Model file for the job. Use its own axes, mm. Face numbers are marked on the shaded views. Give positions to 0.01 mm unless a question says otherwise; leave off trailing zeros. Loops run counter-clockwise (first coordinate to the right, second up) from the corner with the lowest first, then second, coordinate; pieces in that order, holes last. Notation, with made-up numbers: (64.25, -15) - (108.25, -15) arc R14 ccw to (108.25, 7) - close; hole circle Ø9 at (5, -26). An arc over 180 degrees is marked (long way). Answer as CSV lines item,"result". Start each with the question number.
Item 1: Pull direction X, two halves, no side cores. Call the marked faces 1, 2 and 3: pulls with the +X half, pulls with the -X half, needs draft (parallel to the pull), parting line crosses it, or undercut.
Item 2: Saw through at C-C on y = 2. Give the cut face in (x, z).
Item 3: Saw through at B-B on z = -18. Give the cut face in (x, y).
Item 4: Drill centre lines: L1, parallel to X at y = 4.25, z = 0; L2, parallel to Z at x = -12, y = 5.75; L3, parallel to Z at x = -5.5, y = 3. Where is each one in solid material? Low to high. Write a range as from..to.
Item 5: Saw through at D-D on z = 3. Give the cut face in (x, y).
Item 6: Saw through at A-A on x = 11.3. Give the cut face in (y, z).
Item 7: Pin check, flat tips, straight feed: pin 1 (4 mm diameter, centred on y = 5, z = -9, fed in from -X); pin 2 (1.5 mm diameter, centred on x = -5.5, z = 17, fed in from -Y); pin 3 (3 mm diameter, centred on y = 5, z = -9, fed in from -X); pin 4 (4.5 mm diameter, centred on y = 5, z = 9, fed in from -X). Stop position of each tip, or through.
from build123d import *

# Parameters (mm, degrees)
SKETCH_1_W          = 32.7
SKETCH_1_H          = 51
EXTRUDE_1_DEPTH     = 12
SKETCH_2_R          = 2.6
SKETCH_2_R_2        = 1.6
CUT_EXTRUDE_1_DEPTH = 33.581781719
SKETCH_3_W          = 10
SKETCH_3_H          = 2
CUT_EXTRUDE_2_DEPTH = 55.884628996


# Read off the part's stored shape, not the designer's step: 高级异型孔1
with BuildPart() as part:
    # 草图1 → 凸台-拉伸1 (new body)
    with BuildSketch(Plane(origin=(0, 0, 0), x_dir=(1, 0, 0), z_dir=(0, 1, 0))):
        Rectangle(SKETCH_1_W, SKETCH_1_H)
    extrude(amount=EXTRUDE_1_DEPTH)

    # 草图2 → 切除-拉伸1 (cut, through all)
    with BuildSketch(Plane(origin=(0, 12, 0), x_dir=(1, 0, 0), z_dir=(0, 1, 0))):
        with Locations(Location((-11.3, 18, 0), (0, 0, 270))):
            Circle(SKETCH_2_R)
        with Locations(Location((11.3, 18, 0), (0, 0, 90))):
            Circle(SKETCH_2_R)
        with Locations(Location((11.3, -18, 0), (0, 0, 270))):
            Circle(SKETCH_2_R)
        with Locations(Location((-11.3, -18, 0), (0, 0, 90))):
            Circle(SKETCH_2_R)
        with Locations(Location((11.3, 0, 0), (0, 0, 270))):
            Circle(SKETCH_2_R_2)
        with Locations(Location((-11.3, 0, 0), (0, 0, 90))):
            Circle(SKETCH_2_R_2)
    extrude(amount=-CUT_EXTRUDE_1_DEPTH, mode=Mode.SUBTRACT)

    # 草图3 → 切除-拉伸2 (cut, through all)
    with BuildSketch(Plane.XY.offset(25.5)):
        with Locations((0, 11)):
            Rectangle(SKETCH_3_W, SKETCH_3_H)
    extrude(amount=-CUT_EXTRUDE_2_DEPTH, mode=Mode.SUBTRACT)

    # 高级异型孔1 outline → 高级异型孔1 (revolve, cut)
    with BuildSketch(Plane(origin=(0, 5, 9), x_dir=(0, 1, 0), z_dir=(0, 0, -1))):
        Polygon((3.6, -16.35), (3.6, -15.35), (2.3, -15.35), (2.3, -5.35), (0, -3.96802058), (0, -16.35), align=None)
    other_1 = revolve(axis=Axis((0, 5, 9), (1, 0, 0)), mode=Mode.SUBTRACT)

    # Other 1 2 outline → Other 1 2 (revolve, cut)
    with BuildSketch(Plane(origin=(0, 5, -9), x_dir=(0, 1, 0), z_dir=(0, 0, -1))):
        Polygon((0, -16.35), (3.6, -16.35), (3.6, -15.35), (2.3, -15.35), (2.3, -5.35), (0, -3.96802058), align=None)
    other_1_2 = revolve(axis=Axis((0, 5, -9), (1, 0, 0)), mode=Mode.SUBTRACT)

    # 镜向1: 高级异型孔1, Other 1 2 across plane
    add(other_1.mirror(Plane(origin=(0, 0, 0), x_dir=(0, 0, 1), z_dir=(1, 0, 0))), mode=Mode.SUBTRACT)
    add(other_1_2.mirror(Plane(origin=(0, 0, 0), x_dir=(0, 0, 1), z_dir=(1, 0, 0))), mode=Mode.SUBTRACT)


solid = part.part
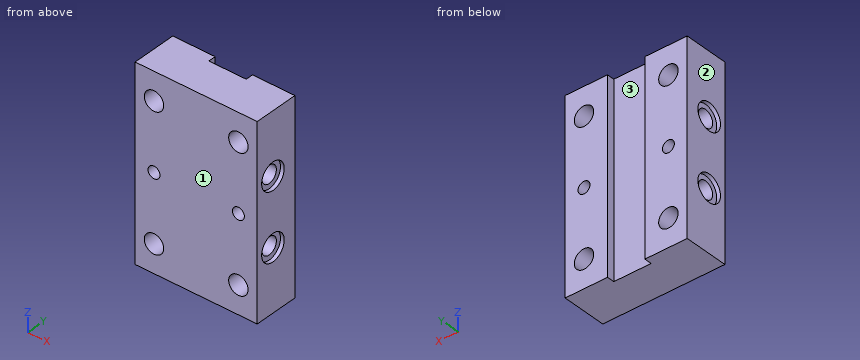
Responses:
1,face 1,"needs draft"
1,face 2,"pulls with the -X half"
1,face 3,"undercut"
2,outline,"(-16.35, -25.5) - (16.35, -25.5) - (16.35, -10.99) - (15.35, -10.99) - (15.35, -7.01) - (16.35, -7.01) - (16.35, 7.01) - (15.35, 7.01) - (15.35, 10.99) - (16.35, 10.99) - (16.35, 25.5) - (-16.35, 25.5) - (-16.35, 10.99) - (-15.35, 10.99) - (-15.35, 7.01) - (-16.35, 7.01) - (-16.35, -7.01) - (-15.35, -7.01) - (-15.35, -10.99) - (-16.35, -10.99) - close; hole circle Ø5.2 at (-11.3, -18); hole circle Ø5.2 at (-11.3, 18); hole circle Ø3.2 at (-11.3, 0); hole circle Ø5.2 at (11.3, -18); hole circle Ø5.2 at (11.3, 18); hole circle Ø3.2 at (11.3, 0)"
3,outline,"(-16.35, 0) - (-13.9, 0) - (-13.9, 12) - (-16.35, 12) - close; (-8.7, 0) - (8.7, 0) - (8.7, 12) - (5, 12) - (5, 10) - (-5, 10) - (-5, 12) - (-8.7, 12) - close; (13.9, 0) - (16.35, 0) - (16.35, 12) - (13.9, 12) - close"
4,L1,"-16.35..-12.9, -9.7..9.7, 12.9..16.35"
4,L2,"-25.5..-20.5, -15.5..-11.17, -6.83..-1.44, 1.44..6.83, 11.17..15.5, 20.5..25.5"
4,L3,"-25.5..-10.14, -7.86..7.86, 10.14..25.5"
5,outline,"(-16.35, 0) - (16.35, 0) - (16.35, 12) - (5, 12) - (5, 10) - (-5, 10) - (-5, 12) - (-16.35, 12) - close"
6,outline,"(0, -25.5) - (12, -25.5) - (12, -20.6) - (0, -20.6) - close; (0, -15.4) - (12, -15.4) - (12, -1.6) - (0, -1.6) - close; (0, 1.6) - (12, 1.6) - (12, 15.4) - (0, 15.4) - close; (0, 20.6) - (12, 20.6) - (12, 25.5) - (0, 25.5) - close; hole circle Ø4.6 at (5, -9); hole circle Ø4.6 at (5, 9)"
7,pin 1,"x = -5.17"
7,pin 2,"y = 0"
7,pin 3,"x = -4.87"
7,pin 4,"x = -5.32"
